from build123d import *

# Parameters (mm, degrees)
F1_DEPTH = 5


with BuildPart() as f1:
    # F0 (on Front) → F1 (new body)
    with BuildSketch(Plane.XZ):
        with BuildLine():
            ThreePointArc((4.847286, -1.473153), (4.914051, -1.23226), (4.968852, -0.988366))
            ThreePointArc((4.968852, -0.988366), (5.011556, -0.742066), (5.042059, -0.49396))
            Line((5.042059, -0.49396), (5.888783, -0.363636))
            ThreePointArc((5.888783, -0.363636), (5.897195, -0.181905), (5.9, 0))
            ThreePointArc((5.9, 0), (5.897195, 0.181905), (5.888783, 0.363636))
            Line((5.888783, 0.363636), (5.042059, 0.49396))
            ThreePointArc((5.042059, 0.49396), (5.011556, 0.742066), (4.968852, 0.988366))
            ThreePointArc((4.968852, 0.988366), (4.914051, 1.23226), (4.847286, 1.473153))
            Line((4.847286, 1.473153), (5.579684, 1.917584))
            ThreePointArc((5.579684, 1.917584), (5.51791, 2.088701), (5.450889, 2.257832))
            ThreePointArc((5.450889, 2.257832), (5.378686, 2.424817), (5.301369, 2.589496))
            Line((5.301369, 2.589496), (4.469225, 2.385872))
            ThreePointArc((4.469225, 2.385872), (4.346098, 2.603419), (4.212389, 2.814629))
            ThreePointArc((4.212389, 2.814629), (4.068426, 3.018985), (3.914557, 3.215992))
            Line((3.914557, 3.215992), (4.421128, 3.906869))
            ThreePointArc((4.421128, 3.906869), (4.298573, 4.041321), (4.17193, 4.17193))
            ThreePointArc((4.17193, 4.17193), (4.041321, 4.298573), (3.906869, 4.421128))
            Line((3.906869, 4.421128), (3.215992, 3.914557))
            ThreePointArc((3.215992, 3.914557), (3.018985, 4.068426), (2.814629, 4.212389))
            ThreePointArc((2.814629, 4.212389), (2.603419, 4.346098), (2.385872, 4.469225))
            Line((2.385872, 4.469225), (2.589496, 5.301369))
            ThreePointArc((2.589496, 5.301369), (2.424817, 5.378686), (2.257832, 5.450889))
            ThreePointArc((2.257832, 5.450889), (2.088701, 5.51791), (1.917584, 5.579684))
            Line((1.917584, 5.579684), (1.473153, 4.847286))
            ThreePointArc((1.473153, 4.847286), (1.23226, 4.914051), (0.988366, 4.968852))
            ThreePointArc((0.988366, 4.968852), (0.742066, 5.011556), (0.49396, 5.042059))
            Line((0.49396, 5.042059), (0.363636, 5.888783))
            ThreePointArc((0.363636, 5.888783), (0.181905, 5.897195), (0, 5.9))
            ThreePointArc((0, 5.9), (-0.181905, 5.897195), (-0.363636, 5.888783))
            Line((-0.363636, 5.888783), (-0.49396, 5.042059))
            ThreePointArc((-0.49396, 5.042059), (-0.742066, 5.011556), (-0.988366, 4.968852))
            ThreePointArc((-0.988366, 4.968852), (-1.23226, 4.914051), (-1.473153, 4.847286))
            Line((-1.473153, 4.847286), (-1.917584, 5.579684))
            ThreePointArc((-1.917584, 5.579684), (-2.088701, 5.51791), (-2.257832, 5.450889))
            ThreePointArc((-2.257832, 5.450889), (-2.424817, 5.378686), (-2.589496, 5.301369))
            Line((-2.589496, 5.301369), (-2.385872, 4.469225))
            ThreePointArc((-2.385872, 4.469225), (-2.603419, 4.346098), (-2.814629, 4.212389))
            ThreePointArc((-2.814629, 4.212389), (-3.018985, 4.068426), (-3.215992, 3.914557))
            Line((-3.215992, 3.914557), (-3.906869, 4.421128))
            ThreePointArc((-3.906869, 4.421128), (-4.041321, 4.298573), (-4.17193, 4.17193))
            ThreePointArc((-4.17193, 4.17193), (-4.298573, 4.041321), (-4.421128, 3.906869))
            Line((-4.421128, 3.906869), (-3.914557, 3.215992))
            ThreePointArc((-3.914557, 3.215992), (-4.068426, 3.018985), (-4.212389, 2.814629))
            ThreePointArc((-4.212389, 2.814629), (-4.346098, 2.603419), (-4.469225, 2.385872))
            Line((-4.469225, 2.385872), (-5.301369, 2.589496))
            ThreePointArc((-5.301369, 2.589496), (-5.378686, 2.424817), (-5.450889, 2.257832))
            ThreePointArc((-5.450889, 2.257832), (-5.51791, 2.088701), (-5.579684, 1.917584))
            Line((-5.579684, 1.917584), (-4.847286, 1.473153))
            ThreePointArc((-4.847286, 1.473153), (-4.914051, 1.23226), (-4.968852, 0.988366))
            ThreePointArc((-4.968852, 0.988366), (-5.011556, 0.742066), (-5.042059, 0.49396))
            Line((-5.042059, 0.49396), (-5.888783, 0.363636))
            ThreePointArc((-5.888783, 0.363636), (-5.897195, 0.181905), (-5.9, 0))
            ThreePointArc((-5.9, 0), (-5.897195, -0.181905), (-5.888783, -0.363636))
            Line((-5.888783, -0.363636), (-5.042059, -0.49396))
            ThreePointArc((-5.042059, -0.49396), (-5.011556, -0.742066), (-4.968852, -0.988366))
            ThreePointArc((-4.968852, -0.988366), (-4.914051, -1.23226), (-4.847286, -1.473153))
            Line((-4.847286, -1.473153), (-5.579684, -1.917584))
            ThreePointArc((-5.579684, -1.917584), (-5.51791, -2.088701), (-5.450889, -2.257832))
            ThreePointArc((-5.450889, -2.257832), (-5.378686, -2.424817), (-5.301369, -2.589496))
            Line((-5.301369, -2.589496), (-4.469225, -2.385872))
            ThreePointArc((-4.469225, -2.385872), (-4.346098, -2.603419), (-4.212389, -2.814629))
            ThreePointArc((-4.212389, -2.814629), (-4.068426, -3.018985), (-3.914557, -3.215992))
            Line((-3.914557, -3.215992), (-4.421128, -3.906869))
            ThreePointArc((-4.421128, -3.906869), (-4.298573, -4.041321), (-4.17193, -4.17193))
            ThreePointArc((-4.17193, -4.17193), (-4.041321, -4.298573), (-3.906869, -4.421128))
            Line((-3.906869, -4.421128), (-3.215992, -3.914557))
            ThreePointArc((-3.215992, -3.914557), (-3.018985, -4.068426), (-2.814629, -4.212389))
            ThreePointArc((-2.814629, -4.212389), (-2.603419, -4.346098), (-2.385872, -4.469225))
            Line((-2.385872, -4.469225), (-2.589496, -5.301369))
            ThreePointArc((-2.589496, -5.301369), (-2.424817, -5.378686), (-2.257832, -5.450889))
            ThreePointArc((-2.257832, -5.450889), (-2.088701, -5.51791), (-1.917584, -5.579684))
            Line((-1.917584, -5.579684), (-1.473153, -4.847286))
            ThreePointArc((-1.473153, -4.847286), (-1.23226, -4.914051), (-0.988366, -4.968852))
            ThreePointArc((-0.988366, -4.968852), (-0.742066, -5.011556), (-0.49396, -5.042059))
            Line((-0.49396, -5.042059), (-0.363636, -5.888783))
            ThreePointArc((-0.363636, -5.888783), (-0.181905, -5.897195), (0, -5.9))
            ThreePointArc((0, -5.9), (0.181905, -5.897195), (0.363636, -5.888783))
            Line((0.363636, -5.888783), (0.49396, -5.042059))
            ThreePointArc((0.49396, -5.042059), (0.742066, -5.011556), (0.988366, -4.968852))
            ThreePointArc((0.988366, -4.968852), (1.23226, -4.914051), (1.473153, -4.847286))
            Line((1.473153, -4.847286), (1.917584, -5.579684))
            ThreePointArc((1.917584, -5.579684), (2.088701, -5.51791), (2.257832, -5.450889))
            ThreePointArc((2.257832, -5.450889), (2.424817, -5.378686), (2.589496, -5.301369))
            Line((2.589496, -5.301369), (2.385872, -4.469225))
            ThreePointArc((2.385872, -4.469225), (2.603419, -4.346098), (2.814629, -4.212389))
            ThreePointArc((2.814629, -4.212389), (3.018985, -4.068426), (3.215992, -3.914557))
            Line((3.215992, -3.914557), (3.906869, -4.421128))
            ThreePointArc((3.906869, -4.421128), (4.041321, -4.298573), (4.17193, -4.17193))
            ThreePointArc((4.17193, -4.17193), (4.298573, -4.041321), (4.421128, -3.906869))
            Line((4.421128, -3.906869), (3.914557, -3.215992))
            ThreePointArc((3.914557, -3.215992), (4.068426, -3.018985), (4.212389, -2.814629))
            ThreePointArc((4.212389, -2.814629), (4.346098, -2.603419), (4.469225, -2.385872))
            Line((4.469225, -2.385872), (5.301369, -2.589496))
            ThreePointArc((5.301369, -2.589496), (5.378686, -2.424817), (5.450889, -2.257832))
            ThreePointArc((5.450889, -2.257832), (5.51791, -2.088701), (5.579684, -1.917584))
            Line((5.579684, -1.917584), (4.847286, -1.473153))
        make_face()
    extrude(amount=F1_DEPTH)


solid = f1.part
For this review, take the finished solid that the model builds, in its own axes (mm). A direction names the side the tool comes from. Coordinates: 2 decimals unless noted, no trailing zeros. Loops run counter-clockwise (first coordinate to the right, second up) from the corner with the lowest first, then second, coordinate; pieces in that order, holes last. Notation, with made-up numbers: (29.5, -23.5) - (66.5, -23.5) arc R17 ccw to (66.5, 1.5) - close; hole circle Ø9 at (28, 33). An arc over 180 degrees is marked (long way). Use a Markdown table: item, result. Add a question column.
Item 1: We need section B-B (z = -0.75). Give the boundary of the cut face in (x, y).
Item 2: Tool access review of faces 1 (the face through (5.47, -2.46, 0.43)), 2 (the face through (4.89, -2.46, 2.49)), 3 (the face through (-4.89, -2.46, -2.49)): name each direction out of +Z, -Z, +X, -X, +Y, -Y from which nothing blocks a thin tool from reaching the whole face with its end or side.
Item 3: Mouldability with a two-part tool opening along X and no side actions: class faces 4 (the face through (4.879, -2.465, -2.486)), 5 (the face through (-5.47, -2.46, -0.43)), 6 (the face through (0, 0, 0)) as pulls with the +X half, pulls with the -X half, needs draft (parallel to the pull), parting line crosses it, or undercut.
Item 4: For line 1 (X direction, y = -3.65, z = -4); line 2 (Z direction, x = -5.25, y = -2.1), list the stretches that pass through material, from the lowest coordinate up.
Item 5: We need section A-A (x = -3.75). Give the boundary of the cut face in (y, z).
Item 6: Insertion check: pin 1 Ø1 at (x, y) = (-3.5, -4) entering from -Z; pin 2 Ø1 at (x, y) = (-3, -3) entering from -Z; pin 3 Ø1.5 at (y, z) = (-3, -2.5) entering from -X. Each pin has a flat end and moves straight along its axis. Give the tip position at first contact, or say it passes through.
Results list:
| question | item | result |
|---|---|---|
| 1 | outline | (-5.01, -5) - (5.01, -5) - (5.01, 0) - (-5.01, 0) - close |
| 2 | face 1 | +X, +Y, -Y |
| 2 | face 2 | +Z, +Y, -Y |
| 2 | face 3 | -Z, +Y, -Y |
| 3 | face 4 | undercut |
| 3 | face 5 | pulls with the -X half |
| 3 | face 6 | needs draft |
| 4 | line 1 | x = -4.34 to -3.33, -3.11 to 3.11, 3.33 to 4.34 |
| 4 | line 2 | z = -2.58 to -1.72, -0.46 to 0.46, 1.72 to 2.58 |
| 5 | outline | (-5, -4.31) - (0, -4.31) - (0, 4.31) - (-5, 4.31) - close |
| 6 | pin 1 | stops at z = -4.42 |
| 6 | pin 2 | stops at z = -5.34 |
| 6 | pin 3 | stops at x = -5.58 |
